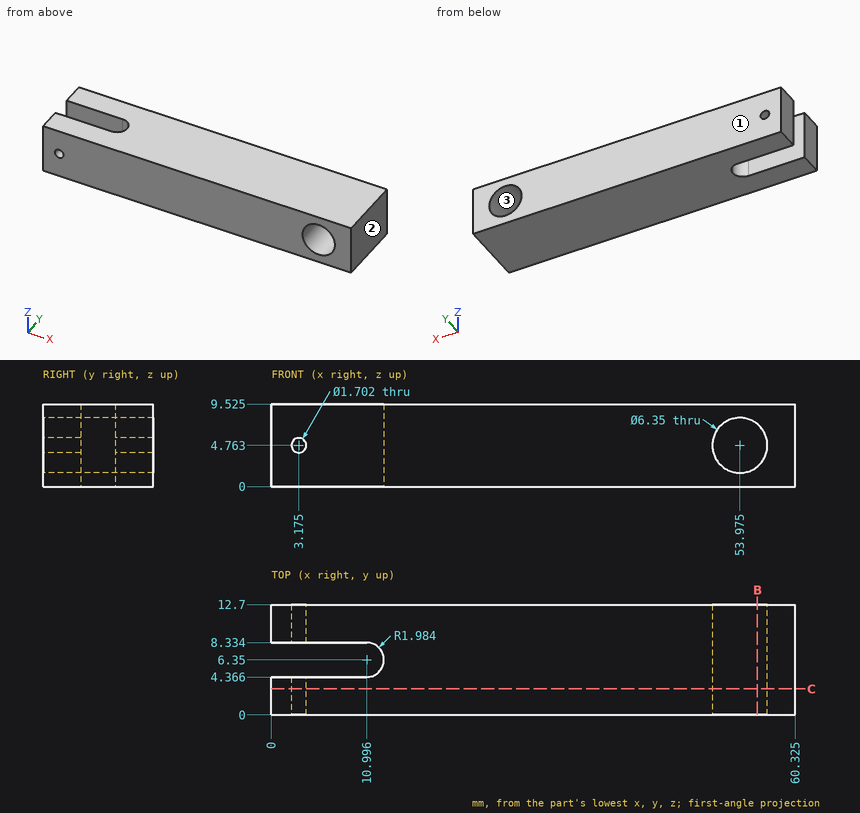
Geometry check sheet. Reference: drawing and pictorial views, mm from the part's lowest x, y, z. Coordinates: 2 decimals unless noted, no trailing zeros. Write each loop counter-clockwise with the first axis right and the second up, starting at its lowest first coordinate (ties: lowest second). Pieces come first, ordered by that corner, then holes. Notation, with made-up numbers: (-9, 5.25) - (35, 5.25) arc R22 cw to (35, 26.25) - close; hole circle Ø6 at (89, -19.5). An arc over 180 degrees is marked (long way). One line per question, with ' | ' between items. Start each with the question number.
1. Section check B-B (x = 56). Enter the section's corners in (y, z) (1 decimal).
2. Material ranges on line 1 along X through (y, z) = (8.75, 5) (1 decimal); line 2 along X through (y, z) = (9.75, 4.25) (1 decimal); line 3 along Y through (x, z) = (10, 8.5), recorded low to high.
3. Draft check along X on the marked faces 1, 2 and 3. Enter one of: released by +X, released by -X, zero draft, split by the parting line, or undercut.
4. Section check C-C (y = 3). Count the separate pieces of the cut face and the enclosed holes in it.
5. Gauge pin test, flat end, axial feed: P1, Ø5.5, axis at x = 53.98, z = 4.76, coming from the -Y side. Record the tip position at first contact, or that the pin passes through.
Computed values:
1) outline: (0, 0) - (12.7, 0) - (12.7, 2.3) - (0, 2.3) - close; (0, 7.2) - (12.7, 7.2) - (12.7, 9.5) - (0, 9.5) - close
2) line 1: 0 to 2.4, 4 to 50.8, 57.1 to 60.3 | line 2: 0 to 2.5, 3.9 to 50.8, 57.1 to 60.3 | line 3: 0 to 4.37, 8.33 to 12.7
3) face 1: zero draft | face 2: released by +X | face 3: undercut
4) separate pieces: 1 | enclosed holes: 2
5) P1: through
